Build history of the part. All positions in model axes, mm. A direction names the side the tool comes from. Round coordinates to 2 decimals unless told otherwise and drop trailing zeros. Write each loop counter-clockwise with the first axis right and the second up, starting at its lowest first coordinate (ties: lowest second). Pieces come first, ordered by that corner, then holes.
Item 1: Wall check: probe 1 along Y at (x, z) = (66.5, 2.2); probe 2 along X at (y, z) = (48.06, 3.35) (3 decimals); probe 3 along X at (y, z) = (70.62, 2.25). Give the ranges that are in metal, low to high.
Item 2: 3-axis set-ups, long thin cutter, end or side, ignore diameter. For faces 1 (the flat face through (-67, 71, 3)), 2 (the cylindrical face through (-68.2, 6.07, 3.85)): which of +Z, -Z, +X, -X, +Y, -Y reach the whole face in a straight line?
Item 3: Drop flat-ended pins along their axis: pin 1 Ø2 at (x, y) = (-61.915, 48.06) entering from -Z; pin 2 Ø4 at (x, y) = (-66.5, 6) entering from -Z; pin 3 Ø5.5 at (x, y) = (0, 92.62) entering from -Z; pin 4 Ø4.5 at (x, y) = (-66.5, 70.62) entering from -Z. Give the stop position or say it passes through.
Item 4: Band-saw the part on A-A, the plane y = 48.06. Write the cut outline in (x, z) (3 decimals).
Item 5: Mould opens along Y. For faces 3 (the flat face through (-69.7, 49, 3)), 4 (the flat face through (1, 2.8, 3)), 5 (the flat face through (-1, 96.32, 3)), 6 (the cylindrical face through (-0.37, 90.96, 3.85)) say: +Y half, -Y half, draft (parallel to the pull), parting line (faces both ways), or undercut.
```python
from build123d import *

# Parameters (mm, degrees)
BOSS_EXTRUDE1_DEPTH                               = 6
SKETCH8_W                                         = 4
SKETCH8_H                                         = 14
SKETCH9_W                                         = 4
SKETCH9_H                                         = 14
SKETCH10_W                                        = 4
SKETCH10_H                                        = 14
SKETCH11_W                                        = 4
SKETCH11_H                                        = 14
CSK_FOR_4_FLAT_HEAD_MACHINE_SCREW_100_D           = 3.4
CSK_FOR_4_FLAT_HEAD_MACHINE_SCREW_100_DEPTH       = 17
CSK_FOR_4_FLAT_HEAD_MACHINE_SCREW_100_CSINK_D     = 6.6
CSK_FOR_4_FLAT_HEAD_MACHINE_SCREW_100_CSINK_ANGLE = 88.289805
F_6_CLEARANCE_HOLE1_D                             = 4.2
F_6_CLEARANCE_HOLE1_DEPTH                         = 6
FILLET2_R                                         = 2.5
SKETCH19_W                                        = 1.65
SKETCH19_H                                        = 6.0002
M4X0_7_TAPPED_HOLE1_AT_2_COUNT                    = 2
M4X0_7_TAPPED_HOLE1_AT_2_PITCH                    = 44.196
M4X0_7_TAPPED_HOLE1_AT_3_COUNT                    = 2
M4X0_7_TAPPED_HOLE1_AT_3_PITCH                    = 131.475918103
M4X0_7_TAPPED_HOLE1_AT_4_COUNT                    = 2
M4X0_7_TAPPED_HOLE1_AT_4_PITCH                    = 123.825
SKETCH20_W                                        = 161.59397274
SKETCH20_H                                        = 68.078942219
CUT_EXTRUDE1_DEPTH                                = 120.401140756


with BuildPart() as part:
    # Sketch1 → Boss-Extrude1 (new body)
    with BuildSketch(Plane(origin=(0, 0, 0), x_dir=(-1, 0, 0), z_dir=(0, 0, -1))):
        with BuildLine():
            Line((-69.7, 93.82), (-69.7, 71.426225775))
            Line((-69.7, 71.426225775), (-69.7, 69.813774225))
            Line((-69.7, 69.813774225), (-69.7, 6.806225775))
            Line((-69.7, 6.806225775), (-69.7, 5.3))
            ThreePointArc((-69.7, 5.3), (-69.699314773, 5.241470835), (-69.69725947, 5.182973755))
            ThreePointArc((-69.69725947, 5.182973755), (-68.967766953, 3.532233047), (-67.317026245, 2.80274053))
            ThreePointArc((-67.317026245, 2.80274053), (-67.258529165, 2.800685227), (-67.2, 2.8))
            Line((-67.2, 2.8), (-65.693774225, 2.8))
            Line((-65.693774225, 2.8), (-0.806225775, 2.8))
            Line((-0.806225775, 2.8), (0.806225775, 2.8))
            Line((0.806225775, 2.8), (65.693774225, 2.8))
            Line((65.693774225, 2.8), (67.2, 2.8))
            ThreePointArc((67.2, 2.8), (67.258529165, 2.800685227), (67.317026245, 2.80274053))
            ThreePointArc((67.317026245, 2.80274053), (68.967766953, 3.532233047), (69.69725947, 5.182973755))
            ThreePointArc((69.69725947, 5.182973755), (69.699314773, 5.241470835), (69.7, 5.3))
            Line((69.7, 5.3), (69.7, 6.806225775))
            Line((69.7, 6.806225775), (69.7, 69.813774225))
            Line((69.7, 69.813774225), (69.7, 71.426225775))
            Line((69.7, 71.426225775), (69.7, 93.82))
            Line((69.7, 93.82), (69.7, 96.32))
            Line((69.7, 96.32), (67.2, 96.32))
            Line((67.2, 96.32), (-67.2, 96.32))
            Line((-67.2, 96.32), (-69.7, 96.32))
            Line((-69.7, 96.32), (-69.7, 93.82))
        make_face()
    extrude(amount=-BOSS_EXTRUDE1_DEPTH)

    # Sketch2 → Cut-Revolve1 (revolve, cut)
    with BuildSketch(Plane(origin=(0, 70.62, 0), x_dir=(1, 0, 0), z_dir=(0, 1, 0)), mode=Mode.PRIVATE) as cut_revolve1_sk:
        Polygon((69.800194118, 0.0002), (66.5, 0.0002), (66.5, -3), (68.2, -3), (68.2, -1.648484848), align=None)
    revolve(cut_revolve1_sk.sketch.rotate(Axis((66.5, 70.62, -0.0002), (0, 0, 1)), 14.141110809), axis=Axis((66.5, 70.62, -0.0002), (0, 0, 1)), mode=Mode.SUBTRACT)

    # Sketch3 → Cut-Revolve2 (revolve, cut)
    with BuildSketch(Plane(origin=(0, 70.62, 0), x_dir=(1, 0, 0), z_dir=(0, 1, 0)), mode=Mode.PRIVATE) as cut_revolve2_sk:
        Polygon((-63.199805882, 0.0002), (-66.5, 0.0002), (-66.5, -3), (-64.8, -3), (-64.8, -1.648484848), align=None)
    revolve(cut_revolve2_sk.sketch.rotate(Axis((-66.5, 70.62, -0.0002), (0, 0, 1)), 165.858889766), axis=Axis((-66.5, 70.62, -0.0002), (0, 0, 1)), mode=Mode.SUBTRACT)

    # Sketch8 → Revolve5 (revolve)
    with BuildSketch(Plane.XZ.offset(-92.256), mode=Mode.PRIVATE) as revolve5_sk:
        with Locations((63.91, 10)):
            Rectangle(SKETCH8_W, SKETCH8_H)
    revolve(revolve5_sk.sketch.rotate(Axis((61.91, 92.256, 17.005), (0, 0, -1)), 180), axis=Axis((61.91, 92.256, 17.005), (0, 0, -1)))

    # Sketch9 → Revolve6 (revolve)
    with BuildSketch(Plane.XZ.offset(-92.256), mode=Mode.PRIVATE) as revolve6_sk:
        with Locations((-59.915, 10)):
            Rectangle(SKETCH9_W, SKETCH9_H)
    revolve(revolve6_sk.sketch.rotate(Axis((-61.915, 92.256, 17.005), (0, 0, -1)), 180), axis=Axis((-61.915, 92.256, 17.005), (0, 0, -1)))

    # Sketch10 → Revolve7 (revolve)
    with BuildSketch(Plane.XZ.offset(-48.06), mode=Mode.PRIVATE) as revolve7_sk:
        with Locations((63.91, 10)):
            Rectangle(SKETCH10_W, SKETCH10_H)
    revolve(revolve7_sk.sketch.rotate(Axis((61.91, 48.06, 17.005), (0, 0, -1)), 180), axis=Axis((61.91, 48.06, 17.005), (0, 0, -1)))

    # Sketch11 → Revolve8 (revolve)
    with BuildSketch(Plane.XZ.offset(-48.06), mode=Mode.PRIVATE) as revolve8_sk:
        with Locations((-59.915, 10)):
            Rectangle(SKETCH11_W, SKETCH11_H)
    revolve(revolve8_sk.sketch.rotate(Axis((-61.915, 48.06, 17.005), (0, 0, -1)), 180), axis=Axis((-61.915, 48.06, 17.005), (0, 0, -1)))

    # CSK for #4 Flat Head Machine Screw (100)1
    with Locations(Plane(origin=(0, 0, 0), x_dir=(-1, 0, 0), z_dir=(0, 0, -1))):
        with Locations((66.5, 6), (0, 6), (-66.5, 6), (0, 92.62)):
            CounterSinkHole(CSK_FOR_4_FLAT_HEAD_MACHINE_SCREW_100_D / 2, CSK_FOR_4_FLAT_HEAD_MACHINE_SCREW_100_CSINK_D / 2, depth=CSK_FOR_4_FLAT_HEAD_MACHINE_SCREW_100_DEPTH, counter_sink_angle=CSK_FOR_4_FLAT_HEAD_MACHINE_SCREW_100_CSINK_ANGLE)

    # #6 Clearance Hole1
    with Locations(Plane.XY.offset(17)):
        with Locations((-61.915, 48.06), (61.91, 48.06), (-61.915, 92.256), (61.91, 92.256)):
            Hole(F_6_CLEARANCE_HOLE1_D / 2, depth=F_6_CLEARANCE_HOLE1_DEPTH)

    # Fillet2
    fillet2_edges = [part.edges().sort_by_distance(p)[0] for p in [
        (69.7, 96.32, 3),
        (-69.7, 96.32, 3),
    ]]
    fillet(fillet2_edges, radius=FILLET2_R)

    # Sketch19 → M4x0.7 Tapped Hole1 (revolve, cut)
    with BuildSketch(Plane(origin=(-61.915, 48.06, 6), x_dir=(0, -1, 0), z_dir=(1, 0, 0))):
        with Locations((0.825, 3.0001)):
            Rectangle(SKETCH19_W, SKETCH19_H)
    m4x0_7_tapped_hole1 = revolve(axis=Axis((-61.915, 48.06, 12.35), (0, 0, -1)), mode=Mode.SUBTRACT)

    # M4x0.7 Tapped Hole1 at 2: M4x0.7 Tapped Hole1 ×2
    with Locations(*[(0, i * M4X0_7_TAPPED_HOLE1_AT_2_PITCH, 0) for i in range(1, M4X0_7_TAPPED_HOLE1_AT_2_COUNT)]):
        add(m4x0_7_tapped_hole1, mode=Mode.SUBTRACT)

    # M4x0.7 Tapped Hole1 at 3: M4x0.7 Tapped Hole1 ×2
    with Locations(*[Vector(0.941807456351738, 0.3361528151901589, 0) * (i * M4X0_7_TAPPED_HOLE1_AT_3_PITCH) for i in range(1, M4X0_7_TAPPED_HOLE1_AT_3_COUNT)]):
        add(m4x0_7_tapped_hole1, mode=Mode.SUBTRACT)

    # M4x0.7 Tapped Hole1 at 4: M4x0.7 Tapped Hole1 ×2
    with Locations(*[(i * M4X0_7_TAPPED_HOLE1_AT_4_PITCH, 0, 0) for i in range(1, M4X0_7_TAPPED_HOLE1_AT_4_COUNT)]):
        add(m4x0_7_tapped_hole1, mode=Mode.SUBTRACT)

    # Sketch20 → Cut-Extrude1 (cut, through all)
    with BuildSketch(Plane.XY.offset(6)):
        with Locations((-0.997493659, 67.826602629)):
            Rectangle(SKETCH20_W, SKETCH20_H)
    extrude(amount=CUT_EXTRUDE1_DEPTH, mode=Mode.SUBTRACT)


solid = part.part
```
Results:
1. probe 1: y = 2.8 to 4.3, 7.7 to 68.92, 72.32 to 96.32
1. probe 2: x = -69.7 to -63.565, -60.265 to 60.26, 63.56 to 69.7
1. probe 3: x = -69.7 to -68.2, -64.8 to 64.8, 68.2 to 69.7
2. face 1: -Z
2. face 2: +Z, -Z
3. pin 1: passes through
3. pin 2: stops at z = 1.34
3. pin 3: stops at z = 0.57
3. pin 4: stops at z = 1.08
4. outline: (-69.7, 0) - (-63.565, 0) - (-63.565, 6) - (-69.7, 6) - close; (-60.265, 0) - (60.26, 0) - (60.26, 6) - (-60.265, 6) - close; (63.56, 0) - (69.7, 0) - (69.7, 6) - (63.56, 6) - close
5. face 3: draft
5. face 4: -Y half
5. face 5: +Y half
5. face 6: undercut
